For this review, use the dimensioned drawing (mm, ordinates from the lowest corner) and the shaded views. Coordinates: 2 decimals unless noted, no trailing zeros. Order: outer loops, then holes, each group sorted by start corner. A loop starts at its lowest first (then second) coordinate and runs counter-clockwise, first axis right, second up. Notation, with made-up numbers: M 68,40 L 127,40 A11 cw 127,61 Z; hole C -26,75 d1. An arc over 180 degrees is marked long. Use one line per item in the form item = value. Start each with the question number.
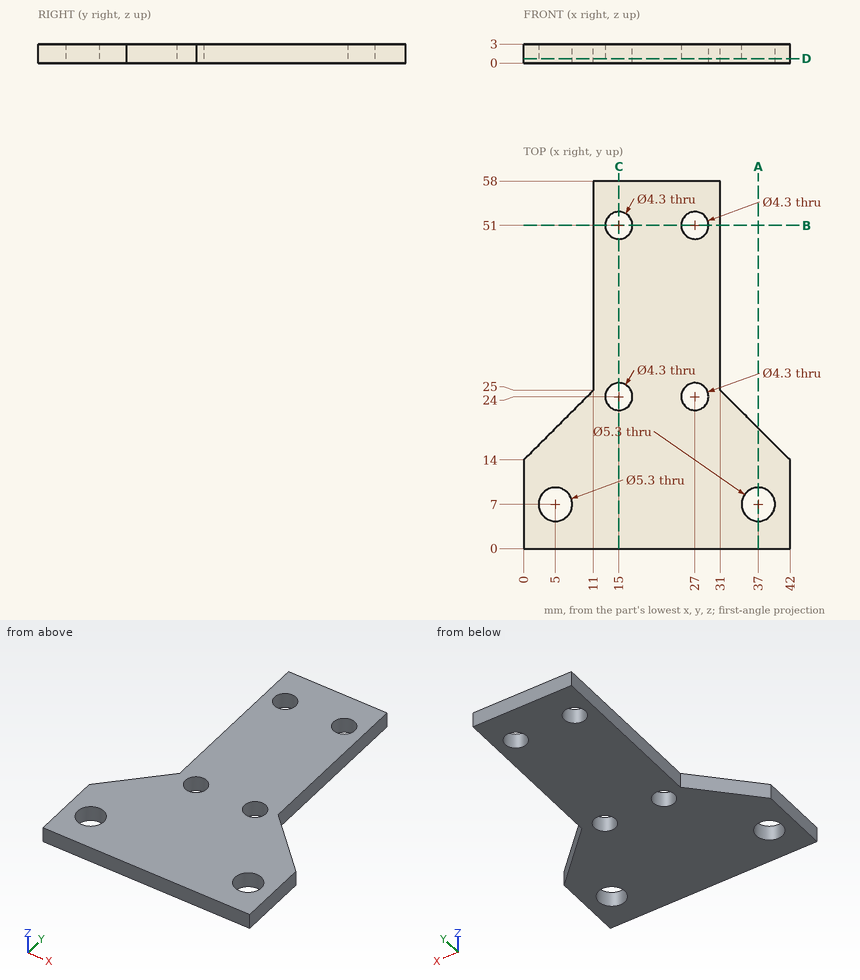
1. To check wall thickness, follow line 1 (X direction, y = 7, z = 0.9); line 2 (X direction, y = 51, z = 1.3); line 3 (Y direction, x = 27, z = 1.3). State the ranges of each line that lie inside material, in increasing order.
2. Consider section D-D, the plane z = 0.7. Write out the cut boundary in (x, y).
3. Consider section B-B, the plane y = 51. Write out the cut boundary in (x, z).
4. For pin 1 Ø8.5 at (x, y) = (37, 7) entering from -Z; pin 2 Ø1.5 at (x, z) = (36, 2) entering from +Y; pin 3 Ø1.5 at (y, z) = (41.5, 1.5) entering from +X; pin 4 Ø4 at (x, y) = (15, 51) entering from +Z, all flat-tipped, find the tip position at first contact; note any pin that passes through.
5. Consider section A-A, the plane x = 37. Write out the cut boundary in (y, z), plus the area to 3 significant figures.
6. Consider section C-C, the plane x = 15. Write out the cut boundary in (y, z), plus the area to 3 significant figures.
Answers follow:
q1.line_1 = 0 to 2.35, 7.65 to 34.35, 39.65 to 42
q1.line_2 = 11 to 12.85, 17.15 to 24.85, 29.15 to 31
q1.line_3 = 0 to 21.85, 26.15 to 48.85, 53.15 to 58
q2.outline = M 0,0 L 42,0 L 42,14 L 31,25 L 31,58 L 11,58 L 11,25 L 0,14 Z; hole C 5,7 d5.3; hole C 15,24 d4.3; hole C 15,51 d4.3; hole C 27,24 d4.3; hole C 27,51 d4.3; hole C 37,7 d5.3
q3.outline = M 11,0 L 12.85,0 L 12.85,3 L 11,3 Z; M 17.15,0 L 24.85,0 L 24.85,3 L 17.15,3 Z; M 29.15,0 L 31,0 L 31,3 L 29.15,3 Z
q4.pin_1 = 0
q4.pin_2 = 20.75
q4.pin_3 = 31
q4.pin_4 = through
q5.outline = M 0,0 L 4.35,0 L 4.35,3 L 0,3 Z; M 9.65,0 L 19,0 L 19,3 L 9.65,3 Z
q5.area = 41.1 mm²
q6.outline = M 0,0 L 21.85,0 L 21.85,3 L 0,3 Z; M 26.15,0 L 48.85,0 L 48.85,3 L 26.15,3 Z; M 53.15,0 L 58,0 L 58,3 L 53.15,3 Z
q6.area = 148 mm²
